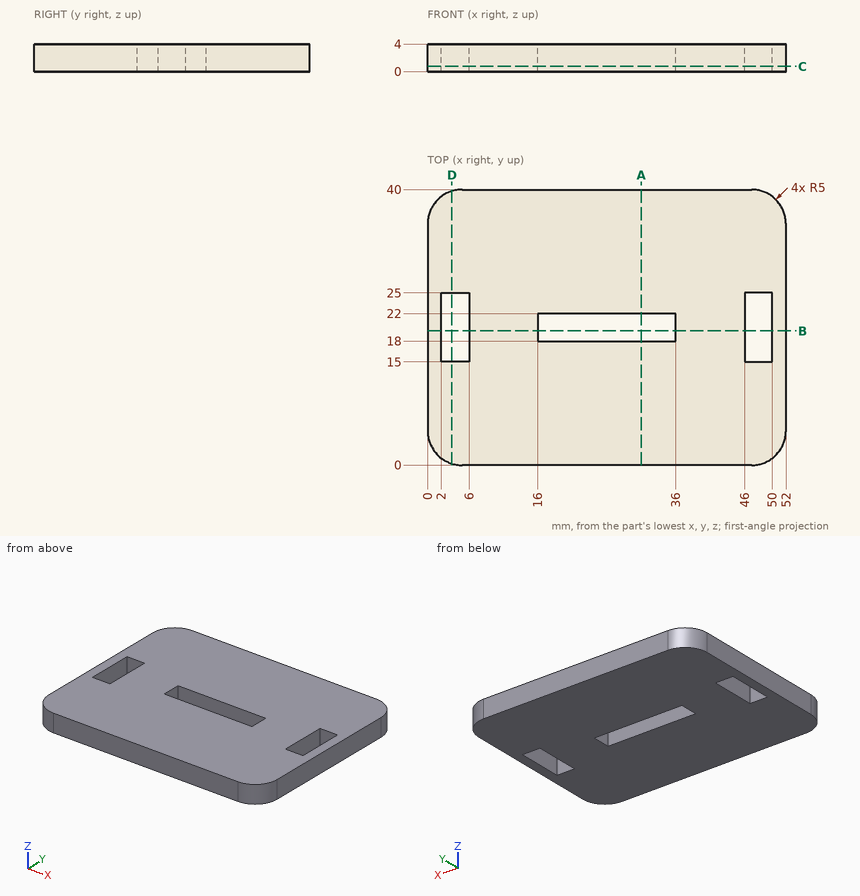
For this review, use the dimensioned drawing (mm, ordinates from the lowest corner) and the shaded views. Coordinates: 2 decimals unless noted, no trailing zeros. Write each loop counter-clockwise with the first axis right and the second up, starting at its lowest first coordinate (ties: lowest second). Pieces come first, ordered by that corner, then holes. Notation, with made-up numbers: (72.5, 72) - (98.5, 72) arc R21 cw to (98.5, 77) - close; hole circle Ø11 at (42, 56). An arc over 180 degrees is marked (long way). One line per item, written item: value.
1) Add section D-D (x = 3.5). State the section outline as (y, z) points.
Answer sheet:
outline: (0.23, 0) - (15, 0) - (15, 4) - (0.23, 4) - close; (25, 0) - (39.77, 0) - (39.77, 4) - (25, 4) - close
2) Add section A-A (x = 31). State the section outline as (y, z) points, plus the area to 3 significant figures.
Answer sheet:
outline: (0, 0) - (18, 0) - (18, 4) - (0, 4) - close; (22, 0) - (40, 0) - (40, 4) - (22, 4) - close
area: 144 mm2
3) Add section B-B (y = 19.5). State the section outline as (x, z) points, plus the area to 3 significant figures.
Answer sheet:
outline: (0, 0) - (2, 0) - (2, 4) - (0, 4) - close; (6, 0) - (16, 0) - (16, 4) - (6, 4) - close; (36, 0) - (46, 0) - (46, 4) - (36, 4) - close; (50, 0) - (52, 0) - (52, 4) - (50, 4) - close
area: 96.0 mm2
4) Add section C-C (z = 0.75). State the section outline as (x, y) points.
Answer sheet:
outline: (0, 5) arc R5 ccw to (5, 0) - (47, 0) arc R5 ccw to (52, 5) - (52, 35) arc R5 ccw to (47, 40) - (5, 40) arc R5 ccw to (0, 35) - close; hole (2, 15) - (6, 15) - (6, 25) - (2, 25) - close; hole (16, 18) - (36, 18) - (36, 22) - (16, 22) - close; hole (46, 15) - (50, 15) - (50, 25) - (46, 25) - close
5) To check wall thickness, follow probe 1 along X at (y, z) = (15.5, 3.25); probe 2 along Y at (x, z) = (31.5, 1.85); probe 3 along X at (y, z) = (21.5, 1.65). State the ranges of each line that lie inside material, in increasing order.
Answer sheet:
probe 1: x = 0 to 2, 6 to 46, 50 to 52
probe 2: y = 0 to 18, 22 to 40
probe 3: x = 0 to 2, 6 to 16, 36 to 46, 50 to 52
6) Insertion check: pin 1 (1.2 mm diameter, centred on x = 4, z = 2, fed in from +Y). The pin has a flat end and moves straight along its axis. Give the tip position at first contact, or say it passes through.
Answer sheet:
pin 1: stops at y = 39.98
